Model file for the job. Use its own axes, mm. A direction names the side the tool comes from. Give positions to 0.01 mm unless a question says otherwise; leave off trailing zeros. Loops run counter-clockwise (first coordinate to the right, second up) from the corner with the lowest first, then second, coordinate; pieces in that order, holes last. Notation, with made-up numbers: M 28,78 L 60,78 A12 cw 60,90 Z; hole C 75,27 d7. An arc over 180 degrees is marked long. Answer in a Markdown table with one row per item.
```python
from build123d import *

# Parameters (mm, degrees)
F0_R     = 9
F1_DEPTH = 1
F2_R     = 2.5
F3_DEPTH = 25


with BuildPart() as f1:
    # F0 (on Top) → F1 (new body)
    with BuildSketch(Plane.XY):
        Circle(F0_R)
    extrude(amount=F1_DEPTH)

    # F2 (on face) → F3 (join)
    with BuildSketch(Plane.XY.offset(1)):
        Circle(F2_R)
    extrude(amount=F3_DEPTH)

    # F5 (on Right) → F6 (revolve, cut)
    with BuildSketch(Plane.YZ):
        Polygon((-2.54262, 21.969934), (-2.54262, 18.685159), (-1.379166, 18.685159), (-1.379166, 20.806479), align=None)
    revolve(axis=Axis((0, 0, 9.517463), (0, 0, 1)), mode=Mode.SUBTRACT)


solid = f1.part
```
(1) Saw through at A-A, the plane y = 0. Give the cut face in (x, z).
Established:
| item | result |
|---|---|
| outline | M -9,0 L 9,0 L 9,1 L 2.5,1 L 2.5,18.69 L 1.38,18.69 L 1.38,20.81 L 2.5,21.93 L 2.5,26 L -2.5,26 L -2.5,21.93 L -1.38,20.81 L -1.38,18.69 L -2.5,18.69 L -2.5,1 L -9,1 Z |
(2) Saw through at C-C, the plane z = 11.5. Give the cut face in (x, y), and give its area (3 significant figures).
Established:
| item | result |
|---|---|
| outline | C 0,0 d5 |
| area | 19.6 mm2 |
(3) Flat gauge pins, fed straight in: P1, Ø3, axis at x = -1, z = 23, coming from the +Y side; P2, Ø6, axis at y = 1, z = 12.5, coming from the +X side; P3, Ø8, axis at x = 5.5, y = 4.5, coming from the +Z side. Where does each tip first touch, or does it go through?
Established:
| item | result |
|---|---|
| P1 | stops at y = 2.5 |
| P2 | stops at x = 2.5 |
| P3 | stops at z = 1 |
(4) Which spindle directions (+Z, -Z, +X, -X, +Y, -Y) get a long thin tool onto all of the face, cutting with end or side? Do faces 1 (the cylindrical face through (-0.54, -2.44, 9.72)), 2 (the flat face through (-1.1, -1.1, 18.685)), 3 (the flat face through (0, 0, 26)). Say none if no direction does.
Established:
| item | result |
|---|---|
| face 1 | +Z |
| face 2 | none |
| face 3 | +Z, +X, -X, +Y, -Y |
(5) Saw through at D-D, the plane x = 7.75. Give the cut face in (y, z), and give its area (3 significant figures).
Established:
| item | result |
|---|---|
| outline | M -4.58,0 L 4.58,0 L 4.58,1 L -4.58,1 Z |
| area | 9.15 mm2 |
(6) Wall check: L1, parallel to Z at x = -4, y = -7.5; L2, parallel to Z at x = 0.75, y = 1.25; L3, parallel to X at y = 1, z = 17. Give the ranges that are in metal, low to high.
Established:
| item | result |
|---|---|
| L1 | z = 0 to 1 |
| L2 | z = 0 to 18.69, 20.89 to 26 |
| L3 | x = -2.29 to 2.29 |
(7) Mould opens along Z. For faces 4 (the cylindrical face through (-1.172, 8.923, 0.493)), 5 (the flat face through (2, -2, 1)), 6 (the cylindrical face through (-1.346, 0.299, 19.761)) say: pulls with the +Z half, pulls with the -Z half, needs draft (parallel to the pull), parting line crosses it, or undercut.
Established:
| item | result |
|---|---|
| face 4 | needs draft |
| face 5 | pulls with the +Z half |
| face 6 | undercut |
